Input: part model. Units: mm. Frame: model coordinates. A direction names the side the tool comes from. Coordinates: 2 decimals unless noted, no trailing zeros. Order: outer loops, then holes, each group sorted by start corner. A loop starts at its lowest first (then second) coordinate and runs counter-clockwise, first axis right, second up. Notation, with made-up numbers: M 30.5,-20.5 L 60.5,-20.5 A30 cw 60.5,7.5 Z; hole C -2.5,-28 d8. An arc over 180 degrees is marked long. Answer in a Markdown table with one row per item.
from build123d import *

# Parameters (mm, degrees)
F0_W      = 200
F0_H      = 30
F1_DEPTH  = 50
F2_W      = 80
F2_H      = 30
F3_DEPTH  = 100
F5_DEPTH  = 25
F6_R      = 3.75
F7_DEPTH  = 70.001
F8_R      = 9.99999
F9_R      = 1
F10_DEPTH = 100.001


# Not quite as in the source:
# - a fillet or chamfer is up to 0.001 mm smaller than in the source, because OpenCascade refuses the exact size


with BuildPart() as f1:
    # F0 (on Right) → F1 (new body, symmetric)
    with BuildSketch(Plane.YZ):
        Rectangle(F0_W, F0_H)
    extrude(amount=F1_DEPTH, both=True)

    # F2 (on face) → F3 (join)
    with BuildSketch(Plane.XY.offset(15)):
        with Locations((0, -85)):
            Rectangle(F2_W, F2_H)
    extrude(amount=F3_DEPTH)

    # F4 (on face) → F5 (join)
    with BuildSketch(Plane.XY.offset(15)):
        Polygon((-20, -40), (-20, -60), (0, -60), (20, -60), (20, -40), align=None)
    extrude(amount=F5_DEPTH)

    # F6 (on face) → F7 (cut, through all)
    with BuildSketch(Plane.YZ.offset(20)):
        with Locations((-50, 30)):
            Circle(F6_R)
    extrude(amount=-F7_DEPTH, mode=Mode.SUBTRACT)

    # F8 (radius 10 in the source; OpenCascade refuses exactly that, so slightly less here)
    f8_edges = [f1.edges().sort_by_distance(p)[0] for p in [
        (0, -40, 40),
        (0, -60, 40),
    ]]
    fillet(f8_edges, radius=F8_R)

    # F9 (on face) → F10 (cut, through all)
    with BuildSketch(Plane.YZ.offset(50)):
        with Locations((90, -5)):
            Circle(F9_R)
        with Locations((-90, -5)):
            Circle(F9_R)
    extrude(amount=-F10_DEPTH, mode=Mode.SUBTRACT)


solid = f1.part
1) Mould query, pull axis Y, two halves, no side actions, for faces 1 (the face through (0, -60, 22)), 2 (the face through (0, -40, 22)), 3 (the face through (50, -1, 0)), 4 (the face through (0.28, -52.764, 32.534)). Classes: +Y half, -Y half, draft (parallel to the pull), parting line (faces both ways), or undercut.
Resolved:
| item | result |
|---|---|
| face 1 | undercut |
| face 2 | +Y half |
| face 3 | draft |
| face 4 | undercut |
2) Cut plane B-B, the plane y = -86. Output: boundary loops of the cut face in (x, z).
Resolved:
| item | result |
|---|---|
| outline | M -50,-15 L 50,-15 L 50,15 L 40,15 L 40,115 L -40,115 L -40,15 L -50,15 Z |
3) Material intervals for probe 1 along Z at (x, y) = (3, 90); probe 2 along Z at (x, y) = (-11.5, -50); probe 3 along Y at (x, z) = (34, 57.5), sorted ascending.
Resolved:
| item | result |
|---|---|
| probe 1 | z = -15 to -6, -4 to 15 |
| probe 2 | z = -15 to 26.25, 33.75 to 40 |
| probe 3 | y = -100 to -70 |
4) Cut plane D-D, the plane z = 65. Output: boundary loops of the cut face in (x, y), and give its area (3 significant figures).
Resolved:
| item | result |
|---|---|
| outline | M -40,-100 L 40,-100 L 40,-70 L -40,-70 Z |
| area | 2,400 mm2 |
5) Contact query for flat-ended pins moving along their axis: pin 1 (24 mm diameter, centred on y = -85, z = 53.5, fed in from -X); pin 2 (3 mm diameter, centred on y = -90, z = -5, fed in from -X); pin 3 (9 mm diameter, centred on y = -79.5, z = 87.5, fed in from +X); pin 4 (1.5 mm diameter, centred on x = -17.5, y = 21, fed in from +Z). Output: stop coordinate, or through.
Resolved:
| item | result |
|---|---|
| pin 1 | stops at x = -40 |
| pin 2 | stops at x = -50 |
| pin 3 | stops at x = 40 |
| pin 4 | stops at z = 15 |
6) Cut plane A-A, the plane x = -7. State how many separate pieces and enclosed holes the cut face has, and give its area (3 significant figures).
Resolved:
| item | result |
|---|---|
| separate pieces | 1 |
| enclosed holes | 3 |
| area | 9,410 mm2 |
7) Cut plane C-C, the plane x = -24.5. Output: boundary loops of the cut face in (y, z), and give its area (3 significant figures).
Resolved:
| item | result |
|---|---|
| outline | M -100,-15 L 100,-15 L 100,15 L -70,15 L -70,115 L -100,115 Z; hole C -90,-5 d2; hole C 90,-5 d2 |
| area | 8,990 mm2 |
8) Reachability of faces 5 (the face through (40, -85, 64)), 6 (the face through (-40, -85, 64)), 7 (the face through (20, -50, 25)), 8 (the face through (-1, -70, 64)) from +Z, -Z, +X, -X, +Y, -Y: full face, straight path, thin tool, end or side. Return the list, or none.
Resolved:
| item | result |
|---|---|
| face 5 | +Z, +X, +Y, -Y |
| face 6 | +Z, -X, +Y, -Y |
| face 7 | +Z, +X, +Y |
| face 8 | +Z, +X, -X |
